```python
from build123d import *

# Parameters (mm, degrees)
BOSS_EXTRUDE1_DEPTH     = 101.6
SHELL1_T                = -12.7
CUT_EXTRUDE1_DEPTH      = 400.9996
CUT_EXTRUDE1_DEPTH_BACK = 400.9996
SKETCH2_W               = 146.165409225
SKETCH2_H               = 51.250950884


with BuildPart() as part:
    # Sketch1 → Boss-Extrude1 (new body)
    with BuildSketch(Plane(origin=(0, 0, 0), x_dir=(1, 0, 0), z_dir=(0, 1, 0))):
        Polygon((-89.538207153, 177.8), (-152.4, 114.938207153), (-152.4, -114.938207153), (-89.538207153, -177.8), (89.538207153, -177.8), (152.4, -114.938207153), (152.4, 114.938207153), (89.538207153, 177.8), align=None)
    extrude(amount=BOSS_EXTRUDE1_DEPTH)

    # Shell1
    shell1_openings = [part.faces().sort_by_distance(p)[0] for p in [
        (0, 101.6, 0),
    ]]
    offset(amount=SHELL1_T, openings=shell1_openings, kind=Kind.INTERSECTION)

    # Sketch2 → Cut-Extrude1 (cut, two sides: drawn at the far end of the back side and taken through both)
    with BuildSketch(Plane.XY.offset(177.8).offset(-CUT_EXTRUDE1_DEPTH_BACK)):
        with Locations((4.47129157, 57.152474053)):
            Rectangle(SKETCH2_W, SKETCH2_H)
    extrude(amount=CUT_EXTRUDE1_DEPTH + CUT_EXTRUDE1_DEPTH_BACK, mode=Mode.SUBTRACT)


solid = part.part
```
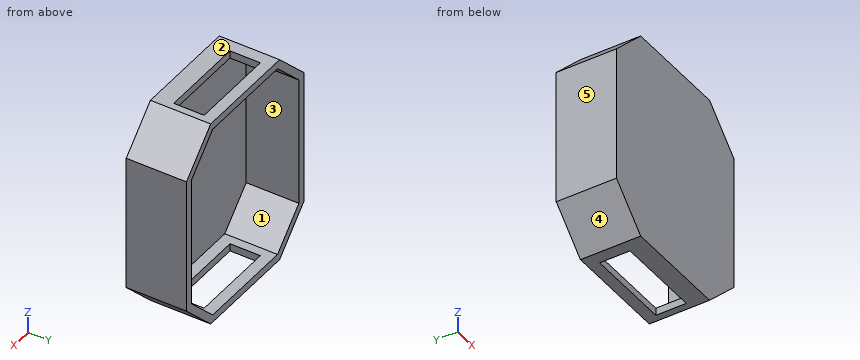
Work out the finished part from the listing and answer in its coordinate system (mm). Face numbers are marked on the shaded views. A direction names the side the tool comes from. Coordinates: 2 decimals unless noted, no trailing zeros. Loops run counter-clockwise (first coordinate to the right, second up) from the corner with the lowest first, then second, coordinate; pieces in that order, holes last. Notation, with made-up numbers: (4.5, 37.5) -> (57.5, 37.5) arc R27 ccw to (57.5, 63.5) -> close; hole circle Ø8 at (34.5, 28). An arc over 180 degrees is marked (long way). Answer as CSV lines item,"result".
Q1. The part is cut by section B-B on y = 72. Write down the section's boundary in (x, z).
Findings:
outline,"(-152.4, -114.94) -> (-89.54, -177.8) -> (-68.61, -177.8) -> (-68.61, -165.1) -> (-84.28, -165.1) -> (-139.7, -109.68) -> (-139.7, 109.68) -> (-84.28, 165.1) -> (-68.61, 165.1) -> (-68.61, 177.8) -> (-89.54, 177.8) -> (-152.4, 114.94) -> close; (77.55, -177.8) -> (89.54, -177.8) -> (152.4, -114.94) -> (152.4, 114.94) -> (89.54, 177.8) -> (77.55, 177.8) -> (77.55, 165.1) -> (84.28, 165.1) -> (139.7, 109.68) -> (139.7, -109.68) -> (84.28, -165.1) -> (77.55, -165.1) -> close"
Q2. A tool of negligible diameter and unlimited length cuts with its end or side. For the marked faces 1 and 2, from which of +Z, -Z, +X, -X, +Y, -Y can it reach the whole face along a straight path? Write none if from no direction.
Findings:
face 1,"+Y"
face 2,"+Z, +X, -X, +Y, -Y"
Q3. For a pull along Z with two mould halves and no side action, classify the marked faces 3, 4 and 5 as +Z half, -Z half, draft (parallel to the pull), parting line (faces both ways), or undercut.
Findings:
face 3,"undercut"
face 4,"-Z half"
face 5,"draft"
Q4. Find the intervals of material crossed by probe 1 along X at (y, z) = (20.5, 41); probe 2 along Z at (x, y) = (-83.5, 17.5); probe 3 along Y at (x, z) = (85, 124.5), in increasing order.
Findings:
probe 1,"x = -152.4 to -139.7, 139.7 to 152.4"
probe 2,"z = -177.8 to -165.1, 165.1 to 177.8"
probe 3,"y = 0 to 12.7"
Q5. The part is cut by section C-C on z = 98. Write down the section's boundary in (x, y).
Findings:
outline,"(-152.4, 0) -> (152.4, 0) -> (152.4, 101.6) -> (139.7, 101.6) -> (139.7, 12.7) -> (-139.7, 12.7) -> (-139.7, 101.6) -> (-152.4, 101.6) -> close"
Q6. The part is cut by section A-A on x = -33.5. Write down the section's boundary in (y, z), and give its area (3 significant figures).
Findings:
outline,"(0, -177.8) -> (31.53, -177.8) -> (31.53, -165.1) -> (12.7, -165.1) -> (12.7, 165.1) -> (31.53, 165.1) -> (31.53, 177.8) -> (0, 177.8) -> close; (82.78, -177.8) -> (101.6, -177.8) -> (101.6, -165.1) -> (82.78, -165.1) -> close; (82.78, 165.1) -> (101.6, 165.1) -> (101.6, 177.8) -> (82.78, 177.8) -> close"
area,"5,470 mm²"
Q7. Each of these flat-tipped pins is pushed along its axis until it touches: pin 1 (10 mm diameter, centred on y = 66, z = -169, fed in from +X); pin 2 (14 mm diameter, centred on y = 44.5, z = -173, fed in from -X); pin 3 (6 mm diameter, centred on x = -101, y = 80, fed in from -Z). Where does it stop, or does it pass through?
Findings:
pin 1,"stops at x = 103.34"
pin 2,"stops at x = -101.34"
pin 3,"stops at z = -169.34"
Q8. The part is cut by section D-D on x = 116.5. Write down the section's boundary in (y, z).
Findings:
outline,"(0, -150.84) -> (101.6, -150.84) -> (101.6, -132.88) -> (12.7, -132.88) -> (12.7, 132.88) -> (101.6, 132.88) -> (101.6, 150.84) -> (0, 150.84) -> close"
